from build123d import *

# Parameters (mm, degrees)
BOSS_EXTRUDE1_DEPTH = 23.5
CUT_EXTRUDE1_DEPTH  = 18
SKETCH3_W           = 7.7
SKETCH3_H           = 25
CUT_EXTRUDE2_DEPTH  = 6.5
SKETCH4_W           = 25
SKETCH4_H           = 7.7
CUT_EXTRUDE3_DEPTH  = 6.5
FILLET1_R           = 2


with BuildPart() as part:
    # Sketch1 → Boss-Extrude1 (new body, symmetric)
    with BuildSketch(Plane.XY):
        Polygon((-47, 0), (0, 0), (0, 47), (-5.5, 47), (-47, 5.5), align=None)
    extrude(amount=BOSS_EXTRUDE1_DEPTH, both=True)

    # Sketch2 → Cut-Extrude1 (cut, symmetric)
    with BuildSketch(Plane.XY):
        Polygon((-5.5, 47), (-5.5, 5.5), (-47, 5.5), align=None)
    extrude(amount=CUT_EXTRUDE1_DEPTH, both=True, mode=Mode.SUBTRACT)

    # Sketch3 → Cut-Extrude2 (cut, through all)
    with BuildSketch(Plane.ZY.offset(5.5)):
        with Locations((0, 28)):
            Rectangle(SKETCH3_W, SKETCH3_H)
    extrude(amount=-CUT_EXTRUDE2_DEPTH, mode=Mode.SUBTRACT)

    # Sketch4 → Cut-Extrude3 (cut, through all)
    with BuildSketch(Plane(origin=(0, 5.5, 0), x_dir=(1, 0, 0), z_dir=(0, 1, 0))):
        with Locations((-25, 0)):
            Rectangle(SKETCH4_W, SKETCH4_H)
    extrude(amount=-CUT_EXTRUDE3_DEPTH, mode=Mode.SUBTRACT)

    # Fillet1
    fillet1_edges = [part.edges().sort_by_distance(p)[0] for p in [
        (-2.75, 47, 23.5),
        (-47, 2.75, 23.5),
        (-2.75, 47, -23.5),
        (-47, 2.75, -23.5),
    ]]
    fillet(fillet1_edges, radius=FILLET1_R)


solid = part.part
Read the model definition and answer for the solid it produces. Units are mm, in the model's axes. A direction names the side the tool comes from. Coordinates: 2 decimals unless noted, no trailing zeros. Loops run counter-clockwise (first coordinate to the right, second up) from the corner with the lowest first, then second, coordinate; pieces in that order, holes last.
Q1. The part is cut by section C-C on z = 15.5. Write down the section's boundary in (x, y).
Q2. Each of these flat-tipped pins is pushed along its axis until it touches: pin 1 Ø1.5 at (y, z) = (21.5, 12) entering from -X; pin 2 Ø4.5 at (x, z) = (-3.5, -1) entering from -Y; pin 3 Ø1.5 at (x, z) = (-36.5, -17) entering from +Y. Where does it stop, or does it pass through?
Q3. The part is cut by section A-A on x = -26. Write down the section's boundary in (y, z).
Q4. The part is cut by section D-D on y = 12. Write down the section's boundary in (x, z).
Q5. The mould has two halves that part along Z. Classify faces 5 (the face through (-3, 28, 3.85)), 6 (the face through (-46.4, 2.86, -22.93)), 7 (the face through (-3, 47, 0)): +Z half, -Z half, draft (parallel to the pull), parting line (faces both ways), or undercut.
Q6. Which of the six approach directions +Z, -Z, +X, -X, +Y, -Y give full straight-line access (tool end or side, diameter ignored) to faces 1 (the face through (-26, 5.5, 4.3)), 2 (the face through (-47, 3, 0)), 3 (the face through (-3, 15.5, 0)), 4 (the face through (-12.5, 3, 0))?
Q7. Consider probe 1 along Z at (x, y) = (-9, 39.5); probe 2 along X at (y, z) = (8, -9); probe 3 along Y at (x, z) = (-41, 17.5). Determine where each line is inside the solid, lowest interval first.
Q8. The part is cut by section B-B on y = 25. Write down the section's boundary in (x, z), and give its area (3 significant figures).
Results below:
1. outline: (-47, 0) - (0, 0) - (0, 47) - (-5.5, 47) - (-5.5, 5.5) - (-47, 5.5) - close
2. pin 1: stops at x = -5.5
2. pin 2: stops at y = 0
2. pin 3: stops at y = 5.5
3. outline: (0, -23.5) - (26.5, -23.5) - (26.5, -18) - (5.5, -18) - (5.5, -3.85) - (0, -3.85) - close; (0, 3.85) - (5.5, 3.85) - (5.5, 18) - (26.5, 18) - (26.5, 23.5) - (0, 23.5) - close
4. outline: (-40.5, -23.5) - (0, -23.5) - (0, 23.5) - (-40.5, 23.5) - (-40.5, 18) - (-5.5, 18) - (-5.5, -18) - (-40.5, -18) - close
5. face 5: undercut
5. face 6: -Z half
5. face 7: draft
6. face 1: -X, +Y
6. face 2: +Z, -Z, -X, +Y, -Y
6. face 3: +X, -X
6. face 4: +Y, -Y
7. probe 1: z = -23.5 to -18, 18 to 23.5
7. probe 2: x = -5.5 to 0
7. probe 3: y = 0 to 5.5
8. outline: (-27.5, -23.5) - (0, -23.5) - (0, -3.85) - (-5.5, -3.85) - (-5.5, -18) - (-27.5, -18) - close; (-27.5, 18) - (-5.5, 18) - (-5.5, 3.85) - (0, 3.85) - (0, 23.5) - (-27.5, 23.5) - close
8. area: 458 mm2
